from build123d import *

# Parameters (mm, degrees)
CROQUIS1_R              = 1.500000001
SALIENTE_EXTRUIR1_DEPTH = 3
CROQUIS4_W              = 3
CROQUIS4_H              = 71.0001277
SALIENTE_EXTRUIR2_DEPTH = 15
CROQUIS5_R              = 6.5
CROQUIS5_R_2            = 1.5
CROQUIS5_R_3            = 2.5
CROQUIS5_W              = 2.499996062
CROQUIS5_H              = 6.000001641
CORTAR_EXTRUIR1_DEPTH   = 10
CORTAR_EXTRUIR3_START   = -3
CORTAR_EXTRUIR3_DEPTH   = 3


# Read off the part's stored shape, not the designer's step: Cortar-Extruir3
with BuildPart() as part:
    # Croquis1 → Saliente-Extruir1 (new body)
    with BuildSketch(Plane.XY):
        with BuildLine():
            Line((314.494178041, 188.579504075), (317.494178043, 188.579506619))
            Line((317.494178043, 188.579506619), (317.494186524, 178.579506615))
            Line((317.494186524, 178.579506615), (314.494177731, 178.579504071))
            Line((314.494177731, 178.579504071), (314.494186212, 168.579504067))
            Line((314.494186212, 168.579504067), (317.494186214, 168.579506611))
            Line((317.494186214, 168.579506611), (317.494190454, 163.579648323))
            Line((317.494190454, 163.579648323), (314.494168474, 163.579645778))
            Line((314.494168474, 163.579645778), (314.494176956, 153.579645774))
            Line((314.494176956, 153.579645774), (317.494159374, 153.579648318))
            Line((317.494159374, 153.579648318), (317.494167855, 143.579648314))
            Line((317.494167855, 143.579648314), (314.494167854, 143.57964577))
            Line((314.494167854, 143.57964577), (314.494173605, 130.579645765))
            Line((314.494173605, 130.579645765), (327.013519861, 130.579618443))
            Line((327.013519861, 130.579618443), (327.013522591, 133.579618444))
            Line((327.013522591, 133.579618444), (339.532765197, 133.579591123))
            Line((339.532765197, 133.579591123), (339.532765197, 130.57943755))
            Line((339.532765197, 130.57943755), (348.284914925, 130.579428178))
            Line((348.284914925, 130.579428178), (348.284918137, 133.579395242))
            Line((348.284918137, 133.579395242), (357.034918141, 133.579385871))
            Line((357.034918141, 133.579385871), (357.034914928, 130.57938587))
            ThreePointArc((357.034914928, 130.57938587), (361.414562849, 127.449962294), (365.794217472, 130.57937649))
            Line((365.794217472, 130.57937649), (365.794220685, 133.579299126))
            Line((365.794220685, 133.579299126), (374.544220688, 133.579289756))
            Line((374.544220688, 133.579289756), (374.544217476, 130.579290106))
            Line((374.544217476, 130.579290106), (383.294100119, 130.579288157))
            Line((383.294100119, 130.579288157), (383.294100787, 133.579288158))
            Line((383.294100787, 133.579288158), (395.694123645, 133.579285396))
            Line((395.694123645, 133.579285396), (395.694122977, 130.579285394))
            Line((395.694122977, 130.579285394), (414.49422245, 130.579281206))
            Line((414.49422245, 130.579281206), (414.494175849, 201.579408906))
            Line((414.494175849, 201.579408906), (395.654796079, 201.579436111))
            Line((395.654796079, 201.579436111), (395.654796079, 198.559911251))
            Line((395.654796079, 198.559911251), (383.254781657, 198.559889448))
            Line((383.254781657, 198.559889448), (383.254781657, 201.579454018))
            Line((383.254781657, 201.579454018), (374.544176149, 201.579466597))
            Line((374.544176149, 201.579466597), (374.544170874, 198.579568646))
            Line((374.544170874, 198.579568646), (365.794170871, 198.579584031))
            Line((365.794170871, 198.579584031), (365.794176145, 201.579506668))
            ThreePointArc((365.794176145, 201.579506668), (361.414530376, 204.708933254), (357.034873601, 201.579522069))
            Line((357.034873601, 201.579522069), (357.034868326, 198.579522068))
            Line((357.034868326, 198.579522068), (348.284868323, 198.579537453))
            Line((348.284868323, 198.579537453), (348.284873598, 201.579504517))
            Line((348.284873598, 201.579504517), (339.493492813, 201.579517212))
            Line((339.493492813, 201.579517212), (339.493492813, 198.559812504))
            Line((339.493492813, 198.559812504), (327.093469951, 198.559790701))
            Line((327.093469951, 198.559790701), (327.093469951, 201.579535118))
            Line((327.093469951, 201.579535118), (314.494181082, 201.579553313))
            Line((314.494181082, 201.579553313), (314.494178041, 188.579504075))
        make_face()
        with Locations((361.414522236, 200.079542161)):
            Circle(CROQUIS1_R, mode=Mode.SUBTRACT)
        with Locations((361.414567806, 132.079353387)):
            Circle(CROQUIS1_R, mode=Mode.SUBTRACT)
    extrude(amount=SALIENTE_EXTRUIR1_DEPTH)

    # Croquis4 → Saliente-Extruir2 (add)
    with BuildSketch(Plane(origin=(414.494308155, 0.000272052, 0), x_dir=(0, 0, -1), z_dir=(0.9999999999997846, 6.563478556519826e-07, 0))):
        with Locations((-1.5, 166.079073004)):
            Rectangle(CROQUIS4_W, CROQUIS4_H)
    extrude(amount=SALIENTE_EXTRUIR2_DEPTH)

    # Croquis5 → Cortar-Extruir1 (cut)
    with BuildSketch(Plane.XY.offset(3)):
        with Locations((398.2941855, 186.875664671)):
            Circle(CROQUIS5_R)
        with Locations((377.694191243, 178.12565115)):
            Circle(CROQUIS5_R_2)
        with Locations((377.694179757, 195.62565115)):
            Circle(CROQUIS5_R_2)
        with Locations((387.4941855, 186.875657583)):
            Circle(CROQUIS5_R_3)
        with Locations((366.2441855, 186.875643636)):
            Rectangle(CROQUIS5_W, CROQUIS5_H)
    extrude(amount=-CORTAR_EXTRUIR1_DEPTH, mode=Mode.SUBTRACT)

    # Cortar-Extruir3 outline → Cortar-Extruir3 (cut)
    with BuildSketch(Plane(origin=(0, 0, 0), x_dir=(-1, 0, 0), z_dir=(0, 0, -1)).offset(CORTAR_EXTRUIR3_START)):
        Polygon((-429.494177993, 198.579387245), (-408.794180476, 198.579417137), (-408.794180476, 201.579419823), (-414.494175849, 201.579408906), (-429.494175849, 201.579418751), align=None)
        Polygon((-408.794229793, 133.579285396), (-429.49422245, 133.579285396), (-429.49422245, 130.579291051), (-414.49422245, 130.579281206), (-408.794229793, 130.579282476), align=None)
    extrude(amount=CORTAR_EXTRUIR3_DEPTH, mode=Mode.SUBTRACT)


solid = part.part
For this review, take the finished solid that the model builds, in its own axes (mm). A direction names the side the tool comes from. Coordinates: 2 decimals unless noted, no trailing zeros. Loops run counter-clockwise (first coordinate to the right, second up) from the corner with the lowest first, then second, coordinate; pieces in that order, holes last. Notation, with made-up numbers: (65.5, 22.5) - (98.5, 22.5) arc R21 ccw to (98.5, 30.5) - close; hole circle Ø5 at (-11.75, 49). An arc over 180 degrees is marked (long way). Use a Markdown table: item, result. Add a question column.
Item 1: Insertion check: pin 1 Ø1.5 at (x, z) = (379.5, 2) entering from +Y; pin 2 Ø1.5 at (x, z) = (331, 2) entering from +Y; pin 3 Ø1.8 at (x, y) = (361.41, 132.08) entering from +Z; pin 4 Ø0.9 at (x, z) = (377.5, 1) entering from -Y. Each pin has a flat end and moves straight along its axis. Give the tip position at first contact, or say it passes through.
Item 2: We need section D-D (y = 146). Give the boundary of the cut face in (x, z), and give its area (3 significant figures).
Item 3: For line 1 (Y direction, x = 362.5, z = 1.75); line 2 (X direction, y = 185.5, z = 1.8); line 3 (Y direction, x = 410, z = 1.05), list the stretches that pass through material, from the lowest coordinate up.
Item 4: Mouldability with a two-part tool opening along Y and no side actions: class faces 6 (the face through (429.494, 167, 2)), 7 (the face through (402, 130.579, 1)), 8 (the face through (316, 178.58, 1)) as pulls with the +Y half, pulls with the -Y half, needs draft (parallel to the pull), parting line crosses it, or undercut.
Item 5: We need section B-B (x = 387). Give the boundary of the cut face in (y, z).
Item 6: We need section A-A (y = 181.5). Give the boundary of the cut face in (x, z).
Item 7: Tool access review of faces 1 (the face through (314.494, 174, 1)), 2 (the face through (339.493, 200, 1)), 3 (the face through (316, 153.58, 1)), 4 (the face through (408.794, 132, 2)), 5 (the face through (383.294, 132, 1)): name each direction out of +Z, -Z, +X, -X, +Y, -Y from which nothing blocks a thin tool from reaching the whole face with its end or side.
Item 8: We need section C-C (z = 0.75). Give the number of separate pieces and of enclosed holes in the cut face, and give its area (3 significant figures).
Results list:
| question | item | result |
|---|---|---|
| 1 | pin 1 | stops at y = 201.58 |
| 1 | pin 2 | stops at y = 198.56 |
| 1 | pin 3 | passes through |
| 1 | pin 4 | stops at y = 130.58 |
| 2 | outline | (317.49, 0) - (429.49, 0) - (429.49, 3) - (317.49, 3) - close |
| 2 | area | 336 mm^2 |
| 3 | line 1 | y = 127.58 to 131.04, 133.11 to 199.04, 201.11 to 204.58 |
| 3 | line 2 | x = 317.49 to 364.99, 367.49 to 385.41, 389.58 to 391.94, 404.65 to 429.49 |
| 3 | line 3 | y = 133.58 to 198.58 |
| 4 | face 6 | needs draft |
| 4 | face 7 | pulls with the -Y half |
| 4 | face 8 | undercut |
| 5 | outline | (133.58, 0) - (184.42, 0) - (184.42, 3) - (133.58, 3) - close; (189.33, 0) - (198.56, 0) - (198.56, 3) - (189.33, 3) - close |
| 6 | outline | (317.49, 0) - (394.64, 0) - (394.64, 3) - (317.49, 3) - close; (401.95, 0) - (429.49, 0) - (429.49, 3) - (401.95, 3) - close |
| 7 | face 1 | +Z, -Z, -X, +Y, -Y |
| 7 | face 2 | +Z, -Z, +Y |
| 7 | face 3 | +Z, -Z, -X |
| 7 | face 4 | +Z, -Z, +X, -Y |
| 7 | face 5 | +Z, -Z, -Y |
| 8 | separate pieces | 1 |
| 8 | enclosed holes | 7 |
| 8 | area | 7,560 mm^2 |
